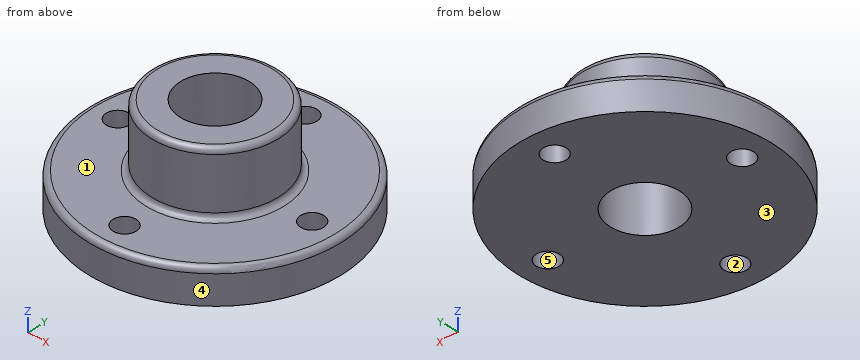
```python
from build123d import *

# Parameters (mm, degrees)
F0_R     = 69.85
F0_R_2   = 6.35
F0_R_3   = 19.05
F1_DEPTH = 19.05
F2_R     = 35.052
F2_R_2   = 19.05
F3_DEPTH = 34.798
F4_R     = 3.048


with BuildPart() as f1:
    # F0 (on Top) → F1 (new body)
    with BuildSketch(Plane.XY):
        Circle(F0_R)
        with Locations((0, -53.848)):
            Circle(F0_R_2, mode=Mode.SUBTRACT)
        with Locations((-53.848, 0)):
            Circle(F0_R_2, mode=Mode.SUBTRACT)
        Circle(F0_R_3, mode=Mode.SUBTRACT)
        with Locations((53.848, 0)):
            Circle(F0_R_2, mode=Mode.SUBTRACT)
        with Locations((0, 53.848)):
            Circle(F0_R_2, mode=Mode.SUBTRACT)
    extrude(amount=F1_DEPTH)

    # F2 (on face) → F3 (join)
    with BuildSketch(Plane.XY.offset(19.05)):
        Circle(F2_R)
        Circle(F2_R_2, mode=Mode.SUBTRACT)
    extrude(amount=F3_DEPTH)

    # F4
    f4_edges = [f1.edges().sort_by_distance(p)[0] for p in [
        (-35.052, 0, 19.05),
        (-35.052, 0, 53.848),
        (-69.85, 0, 19.05),
    ]]
    fillet(f4_edges, radius=F4_R)


solid = f1.part
```
Here's how the part is built. I have some questions about the finished solid (model axes, mm). Face numbers are marked on the shaded views. A direction names the side the tool comes from. Give positions to 0.01 mm unless a question says otherwise; leave off trailing zeros. Write each loop counter-clockwise with the first axis right and the second up, starting at its lowest first coordinate (ties: lowest second). Pieces come first, ordered by that corner, then holes.
(1) Imagine slicing it at C-C, the plane z = 11. Write out the boundary of the cut face in (x, y), and give its area (3 significant figures).
Output values:
outline: circle Ø139.7 at (0, 0); hole circle Ø12.7 at (-53.85, 0); hole circle Ø38.1 at (0, 0); hole circle Ø12.7 at (0, -53.85); hole circle Ø12.7 at (0, 53.85); hole circle Ø12.7 at (53.85, 0)
area: 13,700 mm2
(2) Thinking about a two-plate mould opening in X: for the marked faces 3, 4 and 5, which applies, pulls with the +X half, pulls with the -X half, needs draft (parallel to the pull), parting line crosses it, or undercut?
Output values:
face 3: needs draft
face 4: parting line crosses it
face 5: undercut
(3) Imagine slicing it at D-D, the plane z = 44. Write out the boundary of the cut face in (x, y).
Output values:
outline: circle Ø70.1 at (0, 0); hole circle Ø38.1 at (0, 0)
(4) On a 3-axis mill with a long thin cutter (end or side, diameter ignored), from which of +Z, -Z, +X, -X, +Y, -Y can I reach the whole of each face in a straight line? I mean the marked faces 1 and 2. Say none if no direction works.
Output values:
face 1: +Z
face 2: +Z, -Z
(5) Imagine slicing it at A-A, the plane x = 0. Write out the boundary of the cut face in (y, z).
Output values:
outline: (-69.85, 0) - (-60.2, 0) - (-60.2, 19.05) - (-66.8, 19.05) arc R3.05 ccw to (-69.85, 16) - close; (-47.5, 0) - (-19.05, 0) - (-19.05, 53.85) - (-32, 53.85) arc R3.05 ccw to (-35.05, 50.8) - (-35.05, 22.1) arc R3.05 cw to (-38.1, 19.05) - (-47.5, 19.05) - close; (19.05, 0) - (47.5, 0) - (47.5, 19.05) - (38.1, 19.05) arc R3.05 cw to (35.05, 22.1) - (35.05, 50.8) arc R3.05 ccw to (32, 53.85) - (19.05, 53.85) - close; (60.2, 0) - (69.85, 0) - (69.85, 16) arc R3.05 ccw to (66.8, 19.05) - (60.2, 19.05) - close
(6) If I drill on L1, parallel to Y at x = 0, z = 11; L2, parallel to X at y = -0.5, z = 26; L3, parallel to Z at x = -18, y = -40, over which ranges is the centre line in solid material (lowest first)?
Output values:
L1: y = -69.85 to -60.2, -47.5 to -19.05, 19.05 to 47.5, 60.2 to 69.85
L2: x = -35.05 to -19.04, 19.04 to 35.05
L3: z = 0 to 19.05
(7) Will these pins go through, and if not, where does the flat tip stop? pin 1 (8 mm diameter, centred on y = 16.5, z = 29, fed in from +X); pin 2 (10 mm diameter, centred on x = 0, y = -53.848, fed in from +Z); pin 3 (3 mm diameter, centred on x = -54.5, y = 5.5, fed in from +Z); pin 4 (2 mm diameter, centred on x = -17, z = 25.5, fed in from -Y).
Output values:
pin 1: stops at x = 32.75
pin 2: passes through
pin 3: stops at z = 19.05
pin 4: stops at y = -31.19
